Check sheet for the modelled part. Datum: model origin and axes. Units: mm. A direction names the side the tool comes from. Coordinates: 2 decimals unless noted, no trailing zeros. Loops run counter-clockwise (first coordinate to the right, second up) from the corner with the lowest first, then second, coordinate; pieces in that order, holes last. Notation, with made-up numbers: (41.5, 19) - (89.5, 19) arc R27 ccw to (89.5, 51) - close; hole circle Ø3 at (-13.5, 67). An arc over 180 degrees is marked (long way). Use a Markdown table: item, result. Add a question column.
1) Go/stop test with flat-tipped pins: P1, Ø3, axis at x = -4.5, z = 6.5, coming from the +Y side; P2, Ø6, axis at y = 26, z = 6.5, coming from the +X side; P3, Ø6, axis at x = -15.5, z = 1.5, coming from the +Y side; P4, Ø1, axis at x = 2, y = -12, coming from the +Z side. Record where each tip stops, or that it passes through.
2) Thickness scan on line 1 (X direction, y = 4, z = 4.25); line 2 (X direction, y = -59.5, z = 9.75). Record the ranges inside material, lowest first.
3) Tool access check on faces 5 (the flat face through (0.459, 35, 6)), 6 (the flat face through (-2, 105.498, 6)), 7 (the cylindrical face through (-3.671, 100.568, 4.467)), 8 (the flat face through (-11.97, -52.81, 5.92)), 9 (the flat face through (-14, -34.502, 6)). Record the directions out of +Z, -Z, +X, -X, +Y, -Y that give a thin tool (end or side, any length) a straight path to the whole face; none if there is none.
4) Sectioned sample at B-B, the plane x = -15. Enter the section's corners in (y, z), then the cut area to 3 significant figures.
5) Draft check along X on faces 1 (the flat face through (-9.541, 36, 6)), 2 (the flat face through (-5, 95.498, 6)), 3 (the flat face through (-5, 18, 0)), 4 (the flat face through (2.68, -53.33, 5.92)). Enter one of: pulls with the +X half, pulls with the -X half, needs draft (parallel to the pull), parting line crosses it, or undercut.
6) Sectioned sample at A-A, the plane y = 12. Enter the section's corners in (x, z).
from build123d import *

# Parameters (mm, degrees)
BOSS_EXTRUDE1_DEPTH = 12
SKETCH2_R           = 2
CUT_EXTRUDE1_DEPTH  = 10


with BuildPart() as part:
    # Sketch1 → Boss-Extrude1 (new body)
    with BuildSketch(Plane.XY):
        Polygon((-9.541165506, 105.498159978), (-9.541165506, 95.498159978), (-9.541165506, -34.501840022), (-19.192936941, -34.501840022), (-4.541165506, -71.632080767), (10.110605928, -34.501840022), (0.458834494, -34.501840022), (0.458834494, 95.498159978), (0.458834494, 105.498159978), align=None)
    extrude(amount=BOSS_EXTRUDE1_DEPTH)

    # Sketch2 → Cut-Extrude1 (cut)
    with BuildSketch(Plane(origin=(0, 105.498159978, 0), x_dir=(1, 0, 0), z_dir=(0, 1, 0))):
        with Locations((-4.745886353, -6.153540635)):
            Circle(SKETCH2_R)
    extrude(amount=-CUT_EXTRUDE1_DEPTH, mode=Mode.SUBTRACT)


solid = part.part
Solved:
| question | item | result |
|---|---|---|
| 1 | P1 | stops at y = 95.5 |
| 1 | P2 | stops at x = 0.46 |
| 1 | P3 | stops at y = -34.5 |
| 1 | P4 | passes through |
| 2 | line 1 | x = -9.54 to 0.46 |
| 2 | line 2 | x = -9.33 to 0.25 |
| 3 | face 5 | +Z, -Z, +X, +Y |
| 3 | face 6 | +Z, -Z, +X, -X, +Y |
| 3 | face 7 | +Y |
| 3 | face 8 | +Z, -Z, -X, -Y |
| 3 | face 9 | +Z, -Z, -X, +Y |
| 4 | outline | (-45.13, 0) - (-34.5, 0) - (-34.5, 12) - (-45.13, 12) - close |
| 4 | area | 128 mm2 |
| 5 | face 1 | pulls with the -X half |
| 5 | face 2 | undercut |
| 5 | face 3 | needs draft |
| 5 | face 4 | pulls with the +X half |
| 6 | outline | (-9.54, 0) - (0.46, 0) - (0.46, 12) - (-9.54, 12) - close |
